Input: part model. Units: mm. Frame: model coordinates. Face numbers are marked on the shaded views. A direction names the side the tool comes from. Round coordinates to 2 decimals unless told otherwise and drop trailing zeros. Order: outer loops, then holes, each group sorted by start corner. A loop starts at its lowest first (then second) coordinate and runs counter-clockwise, first axis right, second up. Notation, with made-up numbers: M 36.5,-20.75 L 82.5,-20.75 A23 cw 82.5,2.25 Z; hole C 70,1 d4. An arc over 180 degrees is marked long. One line per question, with ' | ' between items.
```python
from build123d import *

# Parameters (mm, degrees)
ESQUISSE1_W                  = 150
ESQUISSE1_H                  = 120
BOSS_EXTRU_1_DEPTH           = 29
ENL_V_MAT_EXTRU_1_DEPTH      = 28
ENL_V_MAT_EXTRU_2_DEPTH      = 101.329457289
ENL_V_MAT_EXTRU_3_DEPTH      = 101.329457289
ENL_V_MAT_EXTRU_4_DEPTH      = 165.137137784
ENL_V_MAT_EXTRU_4_DEPTH_BACK = 165.137137784
ESQUISSE6_R                  = 5
ENL_V_MAT_EXTRU_6_DEPTH      = 165.137137784
ENL_V_MAT_EXTRU_6_DEPTH_BACK = 165.137137784
ENL_V_MAT_EXTRU_8_DEPTH      = 28
ESQUISSE13_R                 = 1.65
ENL_V_MAT_EXTRU_9_DEPTH      = 10
CONG_1_DEPTH                 = 30
CONG_2_R                     = 15
ESQUISSE14_W                 = 20.617821527
ESQUISSE14_H                 = 6
ENL_V_MAT_EXTRU_10_DEPTH     = 117.86316785
ENL_V_MAT_EXTRU_11_DEPTH     = 10
ENL_V_MAT_EXTRU_14_DEPTH     = 25
CONG_6_R                     = 3
ESQUISSE17_W                 = 39.451580469
ESQUISSE17_H                 = 13
ENL_V_MAT_EXTRU_15_DEPTH     = 22
ESQUISSE18_W                 = 3.388992405
ESQUISSE18_H                 = 13
ENL_V_MAT_EXTRU_16_DEPTH     = 22


with BuildPart() as part:
    # Esquisse1 → Boss.-Extru.1 (new body)
    with BuildSketch(Plane.XY):
        Rectangle(ESQUISSE1_W, ESQUISSE1_H)
    extrude(amount=BOSS_EXTRU_1_DEPTH)

    # Esquisse2 → Enlèv. mat.-Extru.1 (cut)
    with BuildSketch(Plane(origin=(0, 0, 0), x_dir=(-1, 0, 0), z_dir=(0, 0, -1))):
        with BuildLine():
            Line((-13.8, -12), (13.8, -12))
            ThreePointArc((13.8, -12), (16.9, -8.9), (20, -12))
            Line((20, -12), (20, -52))
            ThreePointArc((20, -52), (16.9, -55.1), (13.8, -52))
            Line((13.8, -52), (-13.8, -52))
            ThreePointArc((-13.8, -52), (-16.9, -55.1), (-20, -52))
            Line((-20, -52), (-20, -12))
            ThreePointArc((-20, -12), (-16.9, -8.9), (-13.8, -12))
        make_face()
    extrude(amount=-ENL_V_MAT_EXTRU_1_DEPTH, mode=Mode.SUBTRACT)

    # Esquisse3 → Enlèv. mat.-Extru.2 (cut, through all)
    with BuildSketch(Plane(origin=(0, 0, 0), x_dir=(-1, 0, 0), z_dir=(0, 0, -1))):
        with BuildLine():
            Line((-24, -12), (-75, -12))
            Line((-75, -12), (-75, -60))
            Line((-75, -60), (-21, -60))
            Line((-21, -60), (-21, -15))
            ThreePointArc((-21, -15), (-21.878679656, -12.878679656), (-24, -12))
        make_face()
        with BuildLine():
            Line((24, -12), (75, -12))
            Line((75, -12), (75, -60))
            Line((75, -60), (21, -60))
            Line((21, -60), (21, -15))
            ThreePointArc((21, -15), (21.878679656, -12.878679656), (24, -12))
        make_face()
    extrude(amount=-ENL_V_MAT_EXTRU_2_DEPTH, mode=Mode.SUBTRACT)

    # Esquisse5 → Enlèv. mat.-Extru.3 (cut, through all)
    with BuildSketch(Plane(origin=(0, 0, 0), x_dir=(-1, 0, 0), z_dir=(0, 0, -1))):
        with BuildLine():
            Line((-45, 60), (45, 60))
            Line((45, 60), (45, 3.874810027))
            ThreePointArc((45, 3.874810027), (44.121320344, 1.753489683), (42, 0.874810027))
            Line((42, 0.874810027), (-42, 0.874810027))
            ThreePointArc((-42, 0.874810027), (-44.121320344, 1.753489683), (-45, 3.874810027))
            Line((-45, 3.874810027), (-45, 60))
        make_face()
    extrude(amount=-ENL_V_MAT_EXTRU_3_DEPTH, mode=Mode.SUBTRACT)

    # Esquisse6 → Enlèv. mat.-Extru.4 (cut, two sides: drawn at the far end of the back side and taken through both)
    with BuildSketch(Plane.ZY.offset(75).offset(-ENL_V_MAT_EXTRU_4_DEPTH_BACK)):
        with Locations((8, 19)):
            Circle(ESQUISSE6_R)
    extrude(amount=ENL_V_MAT_EXTRU_4_DEPTH + ENL_V_MAT_EXTRU_4_DEPTH_BACK, mode=Mode.SUBTRACT)

    # Esquisse9 → Enlèv. mat.-Extru.6 (cut, two sides: drawn at the far end of the back side and taken through both)
    with BuildSketch(Plane.ZY.offset(75).offset(-ENL_V_MAT_EXTRU_6_DEPTH_BACK)):
        Polygon((0, 27), (16, 27), (16, -11.5), (29, -11.5), (29, 60), (0, 60), align=None)
    extrude(amount=ENL_V_MAT_EXTRU_6_DEPTH + ENL_V_MAT_EXTRU_6_DEPTH_BACK, mode=Mode.SUBTRACT)

    # Esquisse12 → Enlèv. mat.-Extru.8 (cut)
    with BuildSketch(Plane(origin=(0, 0, 0), x_dir=(-1, 0, 0), z_dir=(0, 0, -1))):
        with BuildLine():
            Line((-69, 27), (-69, 11))
            ThreePointArc((-69, 11), (-68.121320344, 8.878679656), (-66, 8))
            Line((-66, 8), (-54, 8))
            ThreePointArc((-54, 8), (-51.878679656, 8.878679656), (-51, 11))
            Line((-51, 11), (-51, 27))
            Line((-51, 27), (-69, 27))
        make_face()
    enl_v_mat_extru_8 = extrude(amount=-ENL_V_MAT_EXTRU_8_DEPTH, mode=Mode.SUBTRACT)

    # Symétrie1: Enlèv. mat.-Extru.8 across plane
    add(enl_v_mat_extru_8.mirror(Plane(origin=(0, 0, 0), x_dir=(0, 0, 1), z_dir=(1, 0, 0))), mode=Mode.SUBTRACT)

    # Esquisse13 → Enlèv. mat.-Extru.9 (cut)
    with BuildSketch(Plane(origin=(0, 0, 0), x_dir=(-1, 0, 0), z_dir=(0, 0, -1))):
        with Locations((-5.55, -8)):
            Circle(ESQUISSE13_R)
        with Locations((5.55, -8)):
            Circle(ESQUISSE13_R)
        with Locations((-6.55, -56)):
            Circle(ESQUISSE13_R)
        with Locations((5.55, -56)):
            Circle(ESQUISSE13_R)
    extrude(amount=-ENL_V_MAT_EXTRU_9_DEPTH, mode=Mode.SUBTRACT)

    # Congé1: read off the stored shape, not the designer's step
    # Congé1 outline → Congé1 (cut)
    with BuildSketch(Plane.XY):
        with BuildLine():
            Line((-75, -12), (-60, -12))
            ThreePointArc((-60, -12), (-70.606601718, -7.606601718), (-75, 3))
            Line((-75, 3), (-75, -12))
        make_face()
    extrude(amount=CONG_1_DEPTH, mode=Mode.SUBTRACT)

    # Congé2
    cong_2_edges = [part.edges().sort_by_distance(p)[0] for p in [
        (75, -12, 14.5),
    ]]
    fillet(cong_2_edges, radius=CONG_2_R)

    # Esquisse14 → Enlèv. mat.-Extru.10 (cut, through all)
    with BuildSketch(Plane.ZY.offset(21)):
        with Locations((18.691089237, -57)):
            Rectangle(ESQUISSE14_W, ESQUISSE14_H)
    extrude(amount=-ENL_V_MAT_EXTRU_10_DEPTH, mode=Mode.SUBTRACT)

    # Esquisse15 → Enlèv. mat.-Extru.11 (cut)
    with BuildSketch(Plane(origin=(0, -52, 0), x_dir=(1, 0, 0), z_dir=(0, 1, 0))):
        with BuildLine():
            Line((-13.5, -26), (-13.5, -25))
            ThreePointArc((-13.5, -25), (-12.914213562, -23.585786438), (-11.5, -23))
            Line((-11.5, -23), (-6.5, -23))
            ThreePointArc((-6.5, -23), (-5.085786438, -23.585786438), (-4.5, -25))
            Line((-4.5, -25), (-4.5, -26))
            ThreePointArc((-4.5, -26), (-5.085786438, -27.414213562), (-6.5, -28))
            Line((-6.5, -28), (-11.5, -28))
            ThreePointArc((-11.5, -28), (-12.914213562, -27.414213562), (-13.5, -26))
        make_face()
    enl_v_mat_extru_11 = extrude(amount=-ENL_V_MAT_EXTRU_11_DEPTH, mode=Mode.SUBTRACT)

    # Symétrie4: Enlèv. mat.-Extru.11 across plane
    add(enl_v_mat_extru_11.mirror(Plane(origin=(0, 0, 0), x_dir=(0, 0, 1), z_dir=(1, 0, 0))), mode=Mode.SUBTRACT)

    # Esquisse16 → Enlèv. mat.-Extru.14 (cut)
    with BuildSketch(Plane(origin=(0, 0, 0), x_dir=(-1, 0, 0), z_dir=(0, 0, -1))):
        with BuildLine():
            Line((-12, -53), (-7, -53))
            ThreePointArc((-7, -53), (-4.878679656, -52.121320344), (-4, -50))
            Line((-4, -50), (-15, -50))
            ThreePointArc((-15, -50), (-14.121320344, -52.121320344), (-12, -53))
        make_face()
    enl_v_mat_extru_14 = extrude(amount=-ENL_V_MAT_EXTRU_14_DEPTH, mode=Mode.SUBTRACT)

    # Symétrie5: Enlèv. mat.-Extru.14 across plane
    add(enl_v_mat_extru_14.mirror(Plane(origin=(0, 0, 0), x_dir=(0, 0, 1), z_dir=(1, 0, 0))), mode=Mode.SUBTRACT)

    # Congé6
    cong_6_edges = [part.edges().sort_by_distance(p)[0] for p in [
        (-75, 27, 8),
        (-69, 27, 8),
        (-45, 27, 8),
        (-51, 27, 8),
        (75, 27, 8),
        (69, 27, 8),
        (51, 27, 8),
        (45, 27, 8),
    ]]
    fillet(cong_6_edges, radius=CONG_6_R - 0.0001)  # a hair under: the kernel refuses the full size

    # Esquisse17 → Enlèv. mat.-Extru.15 (cut)
    with BuildSketch(Plane(origin=(0, -11.5, 0), x_dir=(1, 0, 0), z_dir=(0, 1, 0))):
        with Locations((44.114782639, -22.5)):
            Rectangle(ESQUISSE17_W, ESQUISSE17_H)
    enl_v_mat_extru_15 = extrude(amount=-ENL_V_MAT_EXTRU_15_DEPTH, mode=Mode.SUBTRACT)

    # Symétrie6: Enlèv. mat.-Extru.15 across plane
    add(enl_v_mat_extru_15.mirror(Plane(origin=(0, 0, 0), x_dir=(0, 0, 1), z_dir=(1, 0, 0))), mode=Mode.SUBTRACT)

    # Esquisse18 → Enlèv. mat.-Extru.16 (cut)
    with BuildSketch(Plane(origin=(0, -11.5, 0), x_dir=(1, 0, 0), z_dir=(0, 1, 0))):
        with Locations((22.694496202, -22.5)):
            Rectangle(ESQUISSE18_W, ESQUISSE18_H)
    enl_v_mat_extru_16 = extrude(amount=-ENL_V_MAT_EXTRU_16_DEPTH, mode=Mode.SUBTRACT)

    # Symétrie7: Enlèv. mat.-Extru.16 across plane
    add(enl_v_mat_extru_16.mirror(Plane(origin=(0, 0, 0), x_dir=(0, 0, 1), z_dir=(1, 0, 0))), mode=Mode.SUBTRACT)


solid = part.part
```
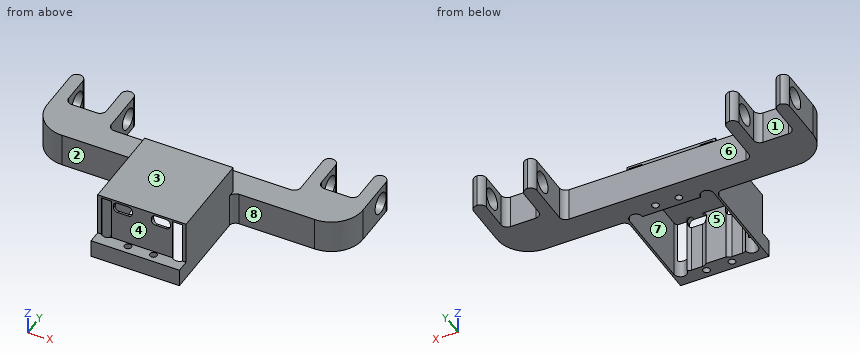
Item 1: Section query B-B, the plane y = -29. Return loops of the section in (x, z), plus the area to 3 significant figures.
Report:
outline: M -21,0 L -20,0 L -20,28 L 20,28 L 20,0 L 21,0 L 21,29 L -21,29 Z | area: 98.0 mm²
Item 2: Section query A-A, the plane x = 16.9. Return loops of the section in (y, z), plus the area to 3 significant figures.
Report:
outline: M -60,0 L -55.1,0 L -55.1,8.38 L -60,8.38 Z; M -54,28 L -11.5,28 L -11.5,29 L -54,29 Z; M -8.9,0 L 0.87,0 L 0.87,16 L -8.9,16 Z | area: 240 mm²
Item 3: Line query: line 1 along Y through (x, z) = (-5.55, 7.5); line 2 along Z through (x, y) = (-73, 19); line 3 along X through (y, z) = (-44, 26.25). Output: solid intervals per line, ascending. Write a range as from..to.
Report:
line 1: -60..-57.65, -54.35..-52.63, -12..-9.65, -6.35..0.87 | line 2: 0..3, 13..16 | line 3: -21..-20, 20..21
Item 4: Section query C-C, the plane x = -35. Return loops of the section in (y, z).
Report:
outline: M -12,0 L 0.87,0 L 0.87,16 L -12,16 Z
Item 5: First-contact query: pin 1 (11.5 mm diameter, centred on y = 19, z = 8, fed in from -X); pin 2 (14 mm diameter, centred on x = -5.5, z = 17, fed in from -Y); pin 3 (6 mm diameter, centred on y = -1.5, z = 5, fed in from +X); pin 4 (10.5 mm diameter, centred on x = -9.5, z = 23, fed in from +Y). Flat tips, straight axial feed; report the tip coordinate or a pass-through.
Report:
pin 1: x = -75 | pin 2: y = -54 | pin 3: x = 74.92 | pin 4: y = -11.5
Item 6: Access query for the marked faces 1, 2, 3 and 4. Directions: +Z, -Z, +X, -X, +Y, -Y. A direction counts if a zero-diameter tool reaches every point of the face in a straight line with its end or side. Return the directions, or none.
Report:
face 1: +Z, -Z, +Y | face 2: +Z, -Z, -X, -Y | face 3: +Z, +X, -X, +Y, -Y | face 4: +Z, +X, -X, -Y
Item 7: Mould query, pull axis Y, two halves, no side actions, for the marked faces 5, 6, 7 and 8. Classes: +Y half, -Y half, draft (parallel to the pull), parting line (faces both ways), or undercut.
Report:
face 5: undercut | face 6: +Y half | face 7: undercut | face 8: -Y half
